Geometry: final body of the model. Coordinates: model frame, mm. A direction names the side the tool comes from. Round coordinates to 2 decimals unless told otherwise and drop trailing zeros. Write each loop counter-clockwise with the first axis right and the second up, starting at its lowest first coordinate (ties: lowest second). Pieces come first, ordered by that corner, then holes. Notation, with made-up numbers: (56.25, 28.5) -> (62.25, 28.5) arc R31 cw to (62.25, 66.5) -> close; hole circle Ø4 at (-37, -5). An arc over 180 degrees is marked (long way). Use one line per item in the form item = value. Start each with the question number.
1. Cut plane D-D, the plane z = -0.75. Return the cut outline in (x, y).
2. Cut plane A-A, the plane z = 3.75. Return the cut outline in (x, y).
3. Draft query along Y for faces 5 (the face through (-16.37, -0.764, -0.068)), 6 (the face through (-3, 0, 0)), 7 (the face through (-17.094, -9, 0)), 8 (the face through (9.8, -15, -0.1)). Return one class per face: pulls with the +Y half, pulls with the -Y half, needs draft (parallel to the pull), parting line crosses it, or undercut.
4. Reachability of faces 1 (the face through (-0.508, 1, 0)), 2 (the face through (0, 1, 0)), 3 (the face through (-25, 5, -1.968)), 4 (the face through (-25, 5, 1.968)) from +Z, -Z, +X, -X, +Y, -Y: full face, straight path, thin tool, end or side. Return the list, or none.
5. Cut plane C-C, the plane y = -8.25. Return the cut outline in (x, z), plus the area to 3 significant figures.
6. Cut plane B-B, the plane x = -9. Return the cut outline in (y, z), plus the area to 3 significant figures.
7. Line query: L1, parallel to Y at x = -5.5, z = -2.5; L2, parallel to Y at x = -16.5, z = -1.75; L3, parallel to X at y = -7, z = 1. Output: solid intervals per line, ascending.
8. Pin query (flat end, axial travel): pin 1 Ø1 at (x, z) = (-14.5, 1.5) entering from +Y; pin 2 Ø0.5 at (x, z) = (11, -1) entering from -Y; pin 3 Ø4 at (x, y) = (-24, 3) entering from -Z. Return the tip coordinate at first contact, or that it passes through.
```python
from build123d import *

# Parameters (mm, degrees)
EXTRUDE_THIN1_DEPTH = 1.9685
SKETCH2_R           = 1.27
BOSS_EXTRUDE1_DEPTH = 4.8895


with BuildPart() as part:
    # Sketch1 → Extrude-Thin1 (new body)
    with BuildSketch(Plane.XY):
        with BuildLine():
            Line((-50.8, 8.3058), (-1.123661277, 2.543344708))
            ThreePointArc((-1.123661277, 2.543344708), (-0.321646116, 2.12650803), (0, 1.281803992))
            Line((0, 1.281803992), (0, 0))
            Line((0, 0), (-0.508, 0))
            Line((-0.508, 0), (-0.508, 1.281803992))
            ThreePointArc((-0.508, 1.281803992), (-0.70098767, 1.788626415), (-1.182196766, 2.038728422))
            Line((-1.182196766, 2.038728422), (-50.858535489, 7.801183714))
            Line((-50.858535489, 7.801183714), (-50.8, 8.3058))
        make_face()
    extrude_thin1 = extrude(amount=-EXTRUDE_THIN1_DEPTH)

    # Sketch2 → Boss-Extrude1 (add)
    with BuildSketch(Plane.XY):
        with BuildLine():
            Line((-14.5542, 0), (9.271, 0))
            ThreePointArc((9.271, 0), (10.169025612, -0.371974388), (10.541, -1.27))
            Line((10.541, -1.27), (10.541, -4.699))
            Line((10.541, -4.699), (11.4808, -4.699))
            Line((11.4808, -4.699), (11.4808, -12.954))
            Line((11.4808, -12.954), (10.541, -12.954))
            Line((10.541, -12.954), (10.541, -13.208))
            ThreePointArc((10.541, -13.208), (9.797051224, -15.004051224), (8.001, -15.748))
            Line((8.001, -15.748), (-15.8242, -15.748))
            ThreePointArc((-15.8242, -15.748), (-16.722225612, -15.376025612), (-17.0942, -14.478))
            Line((-17.0942, -14.478), (-17.0942, -2.54))
            ThreePointArc((-17.0942, -2.54), (-16.350251224, -0.743948776), (-14.5542, 0))
        make_face()
        with Locations((8.001, -2.54)):
            Circle(SKETCH2_R, mode=Mode.SUBTRACT)
        with Locations((-14.5542, -13.208)):
            Circle(SKETCH2_R, mode=Mode.SUBTRACT)
    boss_extrude1 = extrude(amount=-BOSS_EXTRUDE1_DEPTH)

    # Mirror1: Extrude-Thin1, Boss-Extrude1 across Front Plane
    add(extrude_thin1.mirror(Plane.XY))
    add(boss_extrude1.mirror(Plane.XY))


solid = part.part
```
Outcome:
q1.outline = (-50.86, 7.8) -> (-1.18, 2.04) arc R0.76 cw to (-0.51, 1.28) -> (-0.51, 0) -> (-14.55, 0) arc R2.54 ccw to (-17.09, -2.54) -> (-17.09, -14.48) arc R1.27 ccw to (-15.82, -15.75) -> (8, -15.75) arc R2.54 ccw to (10.54, -13.21) -> (10.54, -12.95) -> (11.48, -12.95) -> (11.48, -4.7) -> (10.54, -4.7) -> (10.54, -1.27) arc R1.27 ccw to (9.27, 0) -> (0, 0) -> (0, 1.28) arc R1.27 ccw to (-1.12, 2.54) -> (-50.8, 8.31) -> close; hole circle Ø2.54 at (-14.55, -13.21); hole circle Ø2.54 at (8, -2.54)
q2.outline = (-17.09, -14.48) arc R1.27 ccw to (-15.82, -15.75) -> (8, -15.75) arc R2.54 ccw to (10.54, -13.21) -> (10.54, -12.95) -> (11.48, -12.95) -> (11.48, -4.7) -> (10.54, -4.7) -> (10.54, -1.27) arc R1.27 ccw to (9.27, 0) -> (-14.55, 0) arc R2.54 ccw to (-17.09, -2.54) -> close; hole circle Ø2.54 at (-14.55, -13.21); hole circle Ø2.54 at (8, -2.54)
q3.face_5 = undercut
q3.face_6 = undercut
q3.face_7 = needs draft
q3.face_8 = pulls with the -Y half
q4.face_1 = +Z, -Z, -X
q4.face_2 = +Z, -Z, +X, +Y
q4.face_3 = -Z, +X, -X, +Y
q4.face_4 = +Z, +X, -X, +Y
q5.outline = (-17.09, -4.89) -> (11.48, -4.89) -> (11.48, 4.89) -> (-17.09, 4.89) -> close
q5.area = 279 mm^2
q6.outline = (-15.75, -4.89) -> (0, -4.89) -> (0, 4.89) -> (-15.75, 4.89) -> close; (2.95, -1.97) -> (3.46, -1.97) -> (3.46, 1.97) -> (2.95, 1.97) -> close
q6.area = 156 mm^2
q7.L1 = -15.75 to 0
q7.L2 = -15.55 to -0.91, 3.82 to 4.33
q7.L3 = -17.09 to 11.48
q8.pin_1 = 4.15
q8.pin_2 = -12.95
q8.pin_3 = -1.97
